```python
from build123d import *

# Parameters (mm, degrees)
SKETCH1_R           = 7
BOSS_EXTRUDE1_DEPTH = 30
BOSS_EXTRUDE2_DEPTH = 10


with BuildPart() as part:
    # Sketch1 → Boss-Extrude1 (new body)
    with BuildSketch(Plane.XY):
        Circle(SKETCH1_R)
    extrude(amount=BOSS_EXTRUDE1_DEPTH)

    # Sketch2 → Boss-Extrude2 (add)
    with BuildSketch(Plane.XY.offset(30)):
        with BuildLine():
            Line((3.75, 14.523687548), (31.875, 7.261843774))
            ThreePointArc((31.875, 7.261843774), (37.5, 0), (31.875, -7.261843774))
            Line((31.875, -7.261843774), (3.75, -14.523687548))
            ThreePointArc((3.75, -14.523687548), (-15, 0), (3.75, 14.523687548))
        make_face()
    extrude(amount=BOSS_EXTRUDE2_DEPTH)


solid = part.part
```
CAD build for the part. Positions are in the model's coordinates, mm. A direction names the side the tool comes from. Give positions to 0.01 mm unless a question says otherwise; leave off trailing zeros. Order: outer loops, then holes, each group sorted by start corner. A loop starts at its lowest first (then second) coordinate and runs counter-clockwise, first axis right, second up.
(1) Saw through at C-C, the plane z = 37.5. Give the cut face in (x, y) (3 decimals), then the cut area to 3 significant figures.
(2) Tool access for faces 1 (the cylindrical face through (-15, 0, 35)), 2 (the cylindrical face through (6.466, -2.681, 14.79)): list every direction of +Z, -Z, +X, -X, +Y, -Y with a clear straight run to the whole face (end or side of a thin tool).
(3) Saw through at B-B, the plane x = 0. Give the cut face in (y, z).
(4) Saw through at A-A, the plane y = 0. Give the cut face in (x, z).
(5) Mould opens along Y. For faces 3 (the flat face through (18.01, -10.84, 34.93)), 4 (the flat face through (17.616, 10.944, 34.93)), 5 (the cylindrical face through (37.5, 0.1, 34.9)) say: released by +Y, released by -Y, zero draft, split by the parting line, or undercut.
(6) Flat gauge pins, fed straight in: pin 1 (3 mm diameter, centred on x = 3, z = 6.5, fed in from -Y); pin 2 (1.5 mm diameter, centred on y = 7, z = 13, fed in from +X); pin 3 (6 mm diameter, centred on x = 19.5, y = -4.5, fed in from -Z). Where does each tip first touch, or does it go through?
(7) Saw through at D-D, the plane z = 20. Give the cut face in (x, y).
(8) Drill centre lines: L1, parallel to Z at x = 1, y = -9.25; L2, parallel to X at y = 0.25, z = 33; L3, parallel to X at y = 2, z = 25. Where is each one in solid material? Low to high.
Results found:
1. outline: (3.75, -14.524) - (31.875, -7.262) arc R7.5 ccw to (31.875, 7.262) - (3.75, 14.524) arc R15 ccw (long way) to start
1. area: 1,140 mm2
2. face 1: +Z, -Z
2. face 2: -Z
3. outline: (-15, 30) - (-7, 30) - (-7, 0) - (7, 0) - (7, 30) - (15, 30) - (15, 40) - (-15, 40) - close
4. outline: (-15, 30) - (-7, 30) - (-7, 0) - (7, 0) - (7, 30) - (37.5, 30) - (37.5, 40) - (-15, 40) - close
5. face 3: released by -Y
5. face 4: released by +Y
5. face 5: split by the parting line
6. pin 1: stops at y = -6.84
6. pin 2: stops at x = 3.15
6. pin 3: stops at z = 30
7. outline: circle Ø14 at (0, 0)
8. L1: z = 30 to 40
8. L2: x = -15 to 37.5
8. L3: x = -6.71 to 6.71
